Geometry: see drawing. Coordinates: mm, zero at the bounding-box minimum. A direction names the side the tool comes from. Round coordinates to 2 decimals unless told otherwise and drop trailing zeros. Write each loop counter-clockwise with the first axis right and the second up, starting at its lowest first coordinate (ties: lowest second). Pieces come first, ordered by that corner, then holes. Notation, with made-up numbers: (-37, -22.5) - (3, -22.5) arc R21 cw to (3, -0.5) - close; hole circle Ø5 at (29, -37.75). An arc over 180 degrees is marked (long way). Use a Markdown table: item, result. Add a question column.
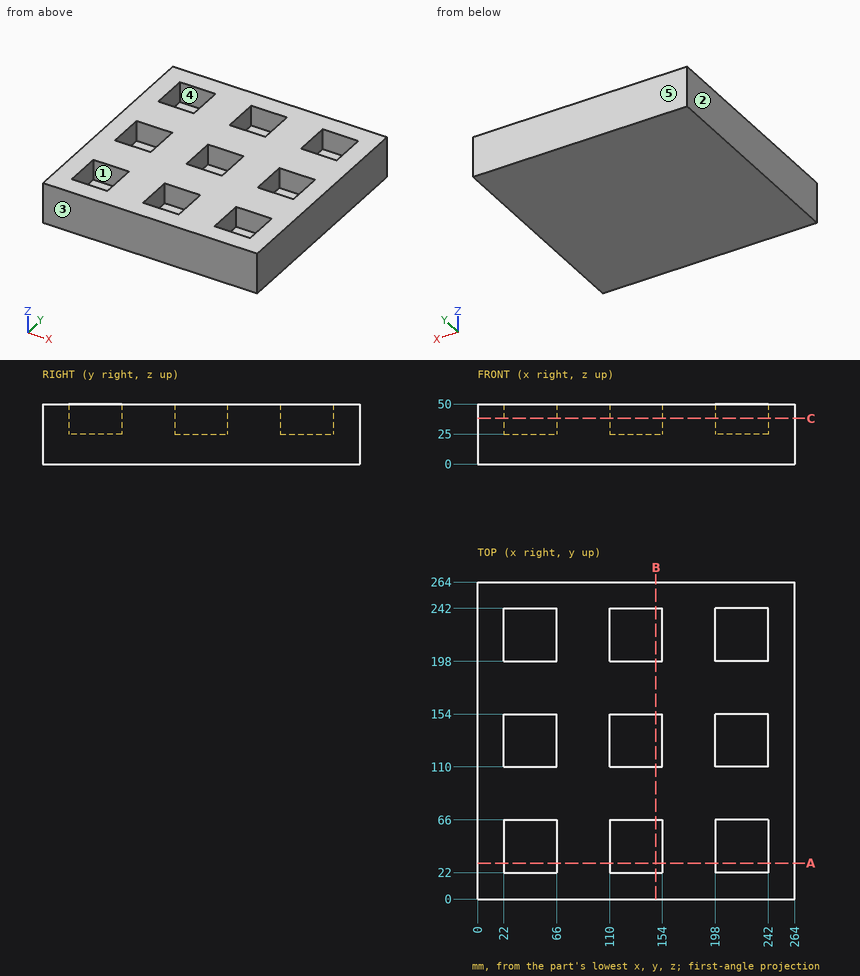
1) Material intervals for L1, parallel to Y at x = 124.5, z = 45.5; L2, parallel to Z at x = 41, y = 139, sorted ascending. Write a range as from..to.
2) Set-up query: the marked faces 4 and 5. Return all of +Z, -Z, +X, -X, +Y, -Y with unobstructed straight access to the full face (end or side cutting, diameter ignored); none if empty.
3) Pin query (flat end, axial travel): P1, Ø22, axis at x = 211.5, y = 213, coming from the +Z side. Return the tip coordinate at first contact, or that it passes through.
4) Section C-C, the plane z = 38. State how many separate pieces and enclosed holes the cut face has, then the cut area to 3 significant figures.
5) Draft query along X for the marked faces 1, 2 and 3. Return one class per face: released by +X, released by -X, zero draft, split by the parting line, or undercut.
6) Section A-A, the plane y = 30. Return the cut outline in (x, z), then the cut area to 3 significant figures.
Output values:
| question | item | result |
|---|---|---|
| 1 | L1 | y = 0..22, 66..110, 154..198, 242..264 |
| 1 | L2 | z = 0..25 |
| 2 | face 4 | +Z |
| 2 | face 5 | +Z, -Z, +X, -X, +Y |
| 3 | P1 | stops at z = 25 |
| 4 | separate pieces | 1 |
| 4 | enclosed holes | 9 |
| 4 | area | 52,300 mm^2 |
| 5 | face 1 | undercut |
| 5 | face 2 | released by -X |
| 5 | face 3 | zero draft |
| 6 | outline | (0, 0) - (264, 0) - (264, 50) - (242, 50) - (242, 25) - (198, 25) - (198, 50) - (154, 50) - (154, 25) - (110, 25) - (110, 50) - (66, 50) - (66, 25) - (22, 25) - (22, 50) - (0, 50) - close |
| 6 | area | 9,900 mm^2 |
